Input: part model. Units: mm. Frame: model coordinates. A direction names the side the tool comes from. Give positions to 0.01 mm unless a question says otherwise; leave off trailing zeros. Loops run counter-clockwise (first coordinate to the right, second up) from the corner with the lowest first, then second, coordinate; pieces in that order, holes last. Notation, with made-up numbers: M 83,-19.75 L 130,-19.75 A22 ccw 130,4.25 Z; hole C 37.5,34 d7. An arc over 180 degrees is marked long. Return JSON: item names as keys, results as strings. Group by question number.
```python
from build123d import *

# Parameters (mm, degrees)
EXTRUDE_2_DEPTH     = 2
SKETCH_4_W          = 2
SKETCH_4_H          = 7
EXTRUDE_3_DEPTH     = 12
FILLET_1_R          = 3.5
SKETCH_5_R          = 1.75
CUT_EXTRUDE_1_DEPTH = 27.177280225
FILLET_2_R          = 3.5
SKETCH_6_R          = 2.75
CUT_EXTRUDE_2_DEPTH = 0.5
CUT_EXTRUDE_START   = -0.5
SKETCH_7_R          = 2.75
CUT_EXTRUDE_3_DEPTH = 0.5


with BuildPart() as part:
    # 草图3 → 凸台-拉伸2 (new body)
    with BuildSketch(Plane.XY):
        with BuildLine():
            Line((-17, -3.5), (-4, -3.5))
            ThreePointArc((-4, -3.5), (0, -1.283009434), (4, -3.5))
            Line((4, -3.5), (17, -3.5))
            Line((17, -3.5), (17, 3.5))
            Line((17, 3.5), (4, 3.5))
            ThreePointArc((4, 3.5), (0, 1.283009434), (-4, 3.5))
            Line((-4, 3.5), (-17, 3.5))
            Line((-17, 3.5), (-17, -3.5))
        make_face()
        with BuildLine():
            Line((-13.5, 1.75), (-8.5, 1.75))
            ThreePointArc((-8.5, 1.75), (-6.75, 0), (-8.5, -1.75))
            Line((-8.5, -1.75), (-13.5, -1.75))
            ThreePointArc((-13.5, -1.75), (-15.25, 0), (-13.5, 1.75))
        make_face(mode=Mode.SUBTRACT)
        with BuildLine():
            Line((13.5, 1.75), (8.5, 1.75))
            ThreePointArc((8.5, 1.75), (6.75, 0), (8.5, -1.75))
            Line((8.5, -1.75), (13.5, -1.75))
            ThreePointArc((13.5, -1.75), (15.25, 0), (13.5, 1.75))
        make_face(mode=Mode.SUBTRACT)
    extrude(amount=EXTRUDE_2_DEPTH)

    # 草图4 → 凸台-拉伸3 (add)
    with BuildSketch(Plane(origin=(0, 0, 0), x_dir=(-1, 0, 0), z_dir=(0, 0, -1))):
        with Locations((-5, 0)):
            Rectangle(SKETCH_4_W, SKETCH_4_H)
        with Locations((5, 0)):
            Rectangle(SKETCH_4_W, SKETCH_4_H)
    extrude(amount=EXTRUDE_3_DEPTH)

    # 圆角1
    fillet_1_edges = [part.edges().sort_by_distance(p)[0] for p in [
        (-5, -3.5, -12),
        (-5, 3.5, -12),
        (5, -3.5, -12),
        (5, 3.5, -12),
    ]]
    fillet(fillet_1_edges, radius=FILLET_1_R - 0.0001)  # a hair under: the kernel refuses the full size

    # 草图5 → 切除-拉伸1 (cut, through all)
    with BuildSketch(Plane(origin=(6, 0, 0), x_dir=(0, 0, -1), z_dir=(1, 0, 0))):
        with Locations(Location((8.5, 0, 0), (0, 0, 270))):
            Circle(SKETCH_5_R)
    extrude(amount=-CUT_EXTRUDE_1_DEPTH, mode=Mode.SUBTRACT)

    # 圆角2
    fillet_2_edges = [part.edges().sort_by_distance(p)[0] for p in [
        (17, -3.5, 1),
        (17, 3.5, 1),
        (-17, -3.5, 1),
        (-17, 3.5, 1),
    ]]
    fillet(fillet_2_edges, radius=FILLET_2_R - 0.0001)  # a hair under: the kernel refuses the full size

    # 草图6 → 切除-拉伸2 (cut)
    with BuildSketch(Plane(origin=(6, 0, 0), x_dir=(0, 0, -1), z_dir=(1, 0, 0))):
        with Locations((8.5, 0)):
            Circle(SKETCH_6_R)
    extrude(amount=-CUT_EXTRUDE_2_DEPTH, mode=Mode.SUBTRACT)

    # 草图7 → 切除-拉伸3 (cut)
    with BuildSketch(Plane.ZY.offset(6).offset(CUT_EXTRUDE_START)):
        with Locations(Location((-8.5, 0, 0), (0, 0, 180))):
            Circle(SKETCH_7_R)
    extrude(amount=CUT_EXTRUDE_3_DEPTH, mode=Mode.SUBTRACT)


solid = part.part
```
Item 1: Material intervals for line 1 (X direction, y = 2, z = -4.75); line 2 (X direction, y = 1.5, z = -10.5); line 3 (Y direction, x = 5.9, z = -8.5), sorted ascending. Write a range as from..to.
Item 2: Section D-D, the plane x = 2.5. Return loops of the section in (y, z), then the cut area to 3 significant figures.
Item 3: Pull-direction query (Z, two-part tool) for faces 6 (the face through (4.76, 0.228, -10.235)), 7 (the face through (-12, 2, 0)), 8 (the face through (15.25, -0.04, 0.99)); classes: pulls with the +Z half, pulls with the -Z half, needs draft (parallel to the pull), parting line crosses it, or undercut.
Item 4: Section C-C, the plane z = -7.5. Return loops of the section in (x, y).
Item 5: First-contact query: pin 1 Ø3.5 at (x, y) = (10, 0.5) entering from -Z; pin 2 Ø3 at (x, z) = (-1.5, -7) entering from +Y; pin 3 Ø4 at (y, z) = (2.5, -8) entering from +X; pin 4 Ø1.6 at (y, z) = (-1, -9) entering from -X. Flat tips, straight axial feed; report the tip coordinate or a pass-through.
Item 6: Reachability of faces 1 (the face through (5.5, -2, -8)), 2 (the face through (-5.5, 2, -8)), 3 (the face through (6.75, 0.04, 0.99)), 4 (the face through (4, 0, -5)), 5 (the face through (6, 0, -5)) from +Z, -Z, +X, -X, +Y, -Y: full face, straight path, thin tool, end or side. Return the list, or none.
Item 7: Section B-B, the plane z = -1. Return loops of the section in (x, y), then the cut area to 3 significant figures.
Item 8: Section A-A, the plane x = 13. Return loops of the section in (y, z).
Answer below:
{
 "1": {"line 1": "-6..-4, 4..6", "line 2": "-5.5..-4, 4..5.5", "line 3": "-3.5..-2.75, 2.75..3.5"},
 "2": {"outline": "M -2,0 L 2,0 L 2,2 L -2,2 Z", "area": "8.00 mm^2"},
 "3": {"face 6": "undercut", "face 7": "pulls with the -Z half", "face 8": "needs draft"},
 "4": {"outline": "M -6,-3.5 L -4,-3.5 L -4,-1.44 L -5.5,-1.44 L -5.5,-2.56 L -6,-2.56 Z; M -6,2.56 L -5.5,2.56 L -5.5,1.44 L -4,1.44 L -4,3.5 L -6,3.5 Z; M 4,-3.5 L 6,-3.5 L 6,-2.56 L 5.5,-2.56 L 5.5,-1.44 L 4,-1.44 Z; M 4,1.44 L 5.5,1.44 L 5.5,2.56 L 6,2.56 L 6,3.5 L 4,3.5 Z"},
 "5": {"pin 1": "z = 0", "pin 2": "through", "pin 3": "x = 6", "pin 4": "x = -5.5"},
 "6": {"face 1": "+X", "face 2": "-X", "face 3": "+Z, -Z", "face 4": "-Z, +Y, -Y", "face 5": "-Z, +X, +Y, -Y"},
 "7": {"outline": "M -6,-3.5 L -4,-3.5 L -4,3.5 L -6,3.5 Z; M 4,-3.5 L 6,-3.5 L 6,3.5 L 4,3.5 Z", "area": "28.0 mm^2"},
 "8": {"outline": "M -3.5,0 L -1.75,0 L -1.75,2 L -3.5,2 Z; M 1.75,0 L 3.5,0 L 3.5,2 L 1.75,2 Z"}
}
